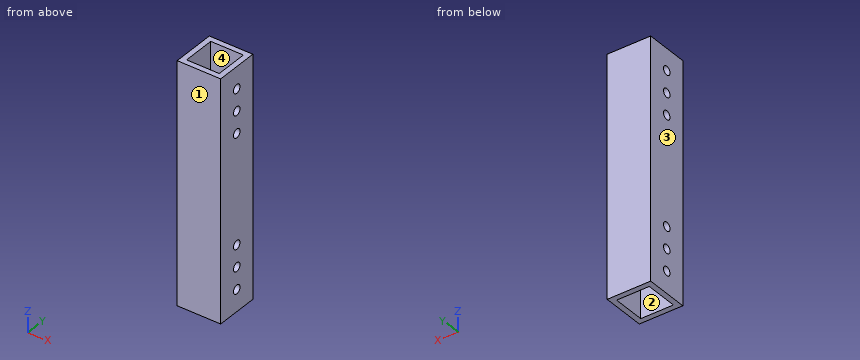
```python
from build123d import *

# Parameters (mm, degrees)
SKETCH1_W              = 25.4
SKETCH1_H              = 25.4
SKETCH1_W_2            = 19.05
SKETCH1_H_2            = 19.05
EXTRUDE_THIN1_DEPTH    = 139.7
F_10_CLEARANCE_HOLE1_D = 5.1054
F_10_CLEARANCE_HOLE2_D = 5.1054


with BuildPart() as part:
    # Sketch1 → Extrude-Thin1 (new body)
    with BuildSketch(Plane.XY):
        with Locations((-12.7, 12.7)):
            Rectangle(SKETCH1_W, SKETCH1_H)
        with Locations((-12.7, 12.7)):
            Rectangle(SKETCH1_W_2, SKETCH1_H_2, mode=Mode.SUBTRACT)
    extrude(amount=EXTRUDE_THIN1_DEPTH)

    # #10 Clearance Hole1 (through all)
    with Locations(Plane(origin=(0, 0, 0), x_dir=(0, 0, -1), z_dir=(1, 0, 0))):
        with Locations((-12.7, 12.7), (-25.4, 12.7), (-38.1, 12.7)):
            Hole(F_10_CLEARANCE_HOLE1_D / 2)

    # #10 Clearance Hole2 (through all)
    with Locations(Plane.ZY.offset(25.4)):
        with Locations((114.3, 12.7), (127, 12.7), (101.6, 12.7)):
            Hole(F_10_CLEARANCE_HOLE2_D / 2)


solid = part.part
```
Model file for the job. Use its own axes, mm. Face numbers are marked on the shaded views. Coordinates: 2 decimals unless noted, no trailing zeros. Order: outer loops, then holes, each group sorted by start corner. A loop starts at its lowest first (then second) coordinate and runs counter-clockwise, first axis right, second up. Notation, with made-up numbers: (-22.5, 50) -> (25.5, 50) arc R19 cw to (25.5, 81) -> close; hole circle Ø5 at (63, 64). An arc over 180 degrees is marked (long way). Answer as a JSON object with one key per item and string values. Group by question number.
1) Cut at B-B, the plane x = -8.25. Write the cut outline in (y, z) (3 decimals).
2) Cut at D-D, the plane z = 76. Write the cut outline in (x, y) (3 decimals), then the cut area to 3 significant figures.
3) Drill centre lines: L1, parallel to Y at x = -15.25, z = 26.5 (3 decimals); L2, parallel to X at y = 19, z = 27 (3 decimals); L3, parallel to Y at x = -1.8, z = 38.1. Where is each one in solid material? Low to high.
4) Flat gauge pins, fed straight in: pin 1 (1.5 mm diameter, centred on x = -20, z = 32, fed in from -Y); pin 2 (4.5 mm diameter, centred on y = 12.7, z = 127, fed in from -X). Where does each tip first touch, or does it go through?
5) Cut at C-C, the plane y = 4.75. Write the cut outline in (x, z) (3 decimals), then the cut area to 3 significant figures.
6) Cut at A-A, the plane z = 127. Write the cut outline in (x, y) (3 decimals).
7) Pull direction Y, two halves, no side cores. Call the marked faces 1, 2, 3 and 4: +Y half, -Y half, draft (parallel to the pull), parting line (faces both ways), or undercut.
Check values:
{
 "1": {"outline": "(0, 0) -> (3.175, 0) -> (3.175, 139.7) -> (0, 139.7) -> close; (22.225, 0) -> (25.4, 0) -> (25.4, 139.7) -> (22.225, 139.7) -> close"},
 "2": {"outline": "(-25.4, 0) -> (0, 0) -> (0, 25.4) -> (-25.4, 25.4) -> close; hole (-22.225, 3.175) -> (-3.175, 3.175) -> (-3.175, 22.225) -> (-22.225, 22.225) -> close", "area": "282 mm²"},
 "3": {"L1": "y = 0 to 3.175, 22.225 to 25.4", "L2": "x = -25.4 to -22.225, -3.175 to 0", "L3": "y = 0 to 10.15, 15.25 to 25.4"},
 "4": {"pin 1": "stops at y = 0", "pin 2": "passes through"},
 "5": {"outline": "(-25.4, 0) -> (-22.225, 0) -> (-22.225, 139.7) -> (-25.4, 139.7) -> close; (-3.175, 0) -> (0, 0) -> (0, 139.7) -> (-3.175, 139.7) -> close", "area": "887 mm²"},
 "6": {"outline": "(-25.4, 0) -> (0, 0) -> (0, 10.147) -> (-3.175, 10.147) -> (-3.175, 3.175) -> (-22.225, 3.175) -> (-22.225, 10.147) -> (-25.4, 10.147) -> close; (-25.4, 15.253) -> (-22.225, 15.253) -> (-22.225, 22.225) -> (-3.175, 22.225) -> (-3.175, 15.253) -> (0, 15.253) -> (0, 25.4) -> (-25.4, 25.4) -> close"},
 "7": {"face 1": "-Y half", "face 2": "undercut", "face 3": "draft", "face 4": "undercut"}
}
